from build123d import *

# Parameters (mm, degrees)
F0_R     = 63.5
F0_R_2   = 6.35
F1_DEPTH = 3.175


# Not quite as in the source:
# - a feature of the source that left no trace in its solid (it failed there, or was rolled back) is left out


with BuildPart() as f1:
    # F0 (on Front) → F1 (new body, symmetric)
    with BuildSketch(Plane.XZ):
        Circle(F0_R)
        with BuildLine():
            ThreePointArc((-6.35, -50.4015624758), (-35.9210244843, -35.9210244843), (-50.4015624758, -6.35))
            Line((-50.4015624758, -6.35), (-17.9605122421, -6.35))
            ThreePointArc((-17.9605122421, -6.35), (-13.4703841816, -13.4703841816), (-6.35, -17.9605122421))
            Line((-6.35, -17.9605122421), (-6.35, -50.4015624758))
        make_face(mode=Mode.SUBTRACT)
        with BuildLine():
            ThreePointArc((50.4015624758, -6.35), (35.9210244843, -35.9210244843), (6.35, -50.4015624758))
            Line((6.35, -50.4015624758), (6.35, -17.9605122421))
            ThreePointArc((6.35, -17.9605122421), (13.4703841816, -13.4703841816), (17.9605122421, -6.35))
            Line((17.9605122421, -6.35), (50.4015624758, -6.35))
        make_face(mode=Mode.SUBTRACT)
        with BuildLine():
            ThreePointArc((-50.4015624758, 6.35), (-35.9210244843, 35.9210244843), (-6.35, 50.4015624758))
            Line((-6.35, 50.4015624758), (-6.35, 17.9605122421))
            ThreePointArc((-6.35, 17.9605122421), (-13.4703841816, 13.4703841816), (-17.9605122421, 6.35))
            Line((-17.9605122421, 6.35), (-50.4015624758, 6.35))
        make_face(mode=Mode.SUBTRACT)
        Circle(F0_R_2, mode=Mode.SUBTRACT)
        with BuildLine():
            Line((50.4015624758, 6.35), (17.9605122421, 6.35))
            ThreePointArc((17.9605122421, 6.35), (13.4703841816, 13.4703841816), (6.35, 17.9605122421))
            Line((6.35, 17.9605122421), (6.35, 50.4015624758))
            ThreePointArc((6.35, 50.4015624758), (35.9210244843, 35.9210244843), (50.4015624758, 6.35))
        make_face(mode=Mode.SUBTRACT)
    extrude(amount=F1_DEPTH, both=True)


solid = f1.part
Read the model definition and answer for the solid it produces. Units are mm, in the model's axes. A direction names the side the tool comes from. Round coordinates to 2 decimals unless told otherwise and drop trailing zeros. Order: outer loops, then holes, each group sorted by start corner. A loop starts at its lowest first (then second) coordinate and runs counter-clockwise, first axis right, second up.
1) Straight lines are drawn through the part: L1, parallel to Z at x = -17, y = -2; L2, parallel to Z at x = 46.5, y = -0.5; L3, parallel to Z at x = 0, y = 0.25. For each, find the intervals that lie inside material, in ascending order.
2) Flat-ended cylindrical pins translate along their axes: pin 1 (1.9 mm diameter, centred on y = -1.5, z = -41.5, fed in from +X); pin 2 (1.9 mm diameter, centred on y = -1.5, z = 34, fed in from -X); pin 3 (2 mm diameter, centred on x = 38.5, y = 2, fed in from -Z). Find the tip coordinate at first contact, or state that the pin passes through.
3) The part is cut by section C-C on z = 0. Write down the section's boundary in (x, y) (3 decimals), plus the area to 3 significant figures.
4) The part is cut by section B-B on x = 0. Write down the section's boundary in (y, z) (3 decimals).
5) For faces 1 (the face through (-13.39, -0.04, 13.55)), 2 (the face through (13, -3.175, 1)), determine the directions among +Z, -Z, +X, -X, +Y, -Y from which every point of the face is accessible in a straight line to the end or side of a thin tool.
6) The part is cut by section D-D on z = -24.5. Write down the section's boundary in (x, y) (3 decimals).
7) The mould has two halves that part along X. Classify faces 3 (the face through (-13.77, -0.04, -61.99)), 4 (the face through (13, 3.175, 1)), 5 (the face through (-35.59, -0.04, -36.25)): released by +X, released by -X, zero draft, split by the parting line, or undercut.
8) The part is cut by section A-A on y = -2. Write down the section's boundary in (x, z).
Resolved:
1. L1: z = -61.18 to -47.87, -8.6 to 8.6, 47.87 to 61.18
1. L2: z = -43.24 to -20.45, -6.35 to 6.35, 20.45 to 43.24
1. L3: z = -63.5 to -6.35, 6.35 to 63.5
2. pin 1: stops at x = 48.87
2. pin 2: stops at x = -54.22
2. pin 3: stops at z = -51.24
3. outline: (-63.5, -3.175) - (-6.35, -3.175) - (-6.35, 3.175) - (-63.5, 3.175) - close; (6.35, -3.175) - (63.5, -3.175) - (63.5, 3.175) - (6.35, 3.175) - close
3. area: 726 mm2
4. outline: (-3.175, -63.5) - (3.175, -63.5) - (3.175, -6.35) - (-3.175, -6.35) - close; (-3.175, 6.35) - (3.175, 6.35) - (3.175, 63.5) - (-3.175, 63.5) - close
5. face 1: +Y, -Y
5. face 2: +Z, -Z, +X, -X, -Y
6. outline: (-58.583, -3.175) - (-44.502, -3.175) - (-44.502, 3.175) - (-58.583, 3.175) - close; (-6.35, -3.175) - (6.35, -3.175) - (6.35, 3.175) - (-6.35, 3.175) - close; (44.502, -3.175) - (58.583, -3.175) - (58.583, 3.175) - (44.502, 3.175) - close
7. face 3: split by the parting line
7. face 4: zero draft
7. face 5: undercut
8. outline: circle Ø127 at (0, 0); hole (-50.4, -6.35) arc R50.8 ccw to (-6.35, -50.4) - (-6.35, -17.96) arc R19.05 cw to (-17.96, -6.35) - close; hole (-50.4, 6.35) - (-17.96, 6.35) arc R19.05 cw to (-6.35, 17.96) - (-6.35, 50.4) arc R50.8 ccw to start; hole circle Ø12.7 at (0, 0); hole (6.35, -50.4) arc R50.8 ccw to (50.4, -6.35) - (17.96, -6.35) arc R19.05 cw to (6.35, -17.96) - close; hole (6.35, 17.96) arc R19.05 cw to (17.96, 6.35) - (50.4, 6.35) arc R50.8 ccw to (6.35, 50.4) - close
